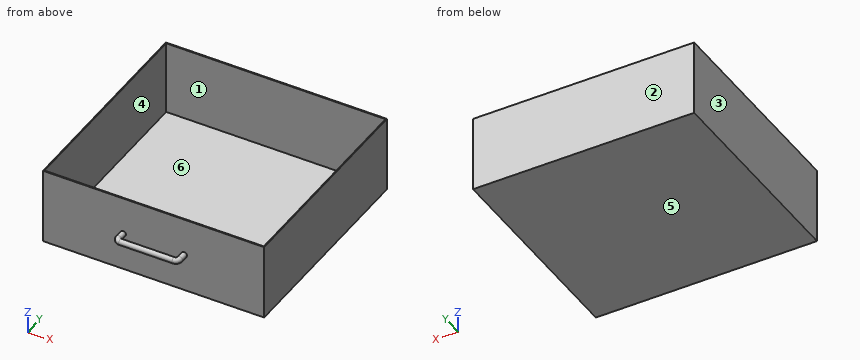
from build123d import *

# Parameters (mm, degrees)
F0_W     = 736.6
F0_H     = 254
F1_DEPTH = 711.2
F2_W     = 730.25
F2_H     = 704.85
F3_DEPTH = 247.65
F5_R     = 9.525


with BuildPart() as f1:
    # F0 (on Front) → F1 (new body)
    with BuildSketch(Plane.XZ):
        Rectangle(F0_W, F0_H)
    extrude(amount=-F1_DEPTH)

    # F2 (on face) → F3 (cut)
    with BuildSketch(Plane.XY.offset(127)):
        with Locations((0, 355.6)):
            Rectangle(F2_W, F2_H)
    extrude(amount=-F3_DEPTH, mode=Mode.SUBTRACT)

    # F6: sweep along a path in F4
    with BuildLine(Plane.XY) as f6_path:
        Line((-101.6, 0), (-101.6, -25.4))
        ThreePointArc((-101.6, -25.4), (-97.8802561211, -34.3802561211), (-88.9, -38.1))
        Line((-88.9, -38.1), (88.9, -38.1))
        ThreePointArc((88.9, -38.1), (97.8802561211, -34.3802561211), (101.6, -25.4))
        Line((101.6, -25.4), (101.6, 0))
    # F5 (on face) → F6 (sweep)
    with BuildSketch(Plane.XZ):
        with Locations((-101.6819179058, 0)):
            Circle(F5_R)
    sweep(path=f6_path.line)


solid = f1.part
Read the model definition and answer for the solid it produces. Units are mm, in the model's axes. Face numbers are marked on the shaded views. A direction names the side the tool comes from. Round coordinates to 2 decimals unless told otherwise and drop trailing zeros. Order: outer loops, then holes, each group sorted by start corner. A loop starts at its lowest first (then second) coordinate and runs counter-clockwise, first axis right, second up. Notation, with made-up numbers: (53.5, 18.25) - (109.5, 18.25) arc R30 ccw to (109.5, 45.25) - close; hole circle Ø9 at (-32, 55). An arc over 180 degrees is marked (long way). Use one line per item in the form item = value. Start each with the question number.
(1) The part is cut by section C-C (y = 132). Give the vertices of the cut face in (x, z) (3 decimals).
(2) The part is cut by section A-A (z = 0). Give the vertices of the cut face in (x, y) (3 decimals).
(3) Determine the mould class of the marked faces 3, 4, 5 and 6 for opening direction X: +X half, -X half, draft (parallel to the pull), parting line (faces both ways), or undercut.
(4) Find the intervals of material crossed by line 1 along X through (y, z) = (43, -75) (3 decimals); line 2 along Y through (x, z) = (294, -23) (3 decimals); line 3 along Z through (x, y) = (-321, 540), in increasing order. Write a range as from..to.
(5) The part is cut by section B-B (x = 69). Give the vertices of the cut face in (y, z) (3 decimals), then the cut area to 3 significant figures.
(6) Flat-ended cylindrical pins translate along their axes: pin 1 Ø2 at (x, z) = (261.5, -75) entering from -Y; pin 2 Ø1.5 at (x, y) = (-289, 202.5) entering from +Z. Find the tip coordinate at first contact, or state that the pin passes through.
(7) The part is cut by section D-D (z = -40). Give the vertices of the cut face in (x, y) (3 decimals).
(8) For the marked faces 1 and 2, determine the directions among +Z, -Z, +X, -X, +Y, -Y from which every point of the face is accessible in a straight line to the end or side of a thin tool.
Checked values:
q1.outline = (-368.3, -127) - (368.3, -127) - (368.3, 127) - (365.125, 127) - (365.125, -120.65) - (-365.125, -120.65) - (-365.125, 127) - (-368.3, 127) - close
q2.outline = (-368.3, 0) - (-111.207, 0) - (-111.207, -25.4) arc R22.307 ccw to (-88.9, -47.707) - (88.9, -47.707) arc R22.307 ccw to (111.207, -25.4) - (111.207, 0) - (368.3, 0) - (368.3, 711.2) - (-368.3, 711.2) - close; hole (-365.125, 3.175) - (365.125, 3.175) - (365.125, 708.025) - (-365.125, 708.025) - close; hole (-92.157, -25.4) arc R3.257 ccw to (-88.9, -28.657) - (88.9, -28.657) arc R3.257 ccw to (92.157, -25.4) - (92.157, 0) - (-92.157, 0) - close
q3.face_3 = -X half
q3.face_4 = undercut
q3.face_5 = draft
q3.face_6 = undercut
q4.line_1 = -368.3..-365.125, 365.125..368.3
q4.line_2 = 0..3.175, 708.025..711.2
q4.line_3 = -127..-120.65
q5.outline = circle Ø19.05 at (-38.182, 0); (0, -127) - (711.2, -127) - (711.2, 127) - (708.025, 127) - (708.025, -120.65) - (3.175, -120.65) - (3.175, 127) - (0, 127) - close
q5.area = 6,370 mm^2
q6.pin_1 = 0
q6.pin_2 = -120.65
q7.outline = (-368.3, 0) - (368.3, 0) - (368.3, 711.2) - (-368.3, 711.2) - close; hole (-365.125, 3.175) - (365.125, 3.175) - (365.125, 708.025) - (-365.125, 708.025) - close
q8.face_1 = +Z
q8.face_2 = +Z, -Z, +X, -X, +Y
